The drawing under review shows one solid part. Ordinate dimensions are in mm from its lowest x, y, z. Coordinates: 2 decimals unless noted, no trailing zeros. Write each loop counter-clockwise with the first axis right and the second up, starting at its lowest first coordinate (ties: lowest second). Pieces come first, ordered by that corner, then holes. Notation, with made-up numbers: (40.5, -5.75) - (91.5, -5.75) arc R8 ccw to (91.5, 3.25) - close; hole circle Ø11 at (23, 58.5). An arc over 180 degrees is marked (long way). Use a Markdown table: item, result.
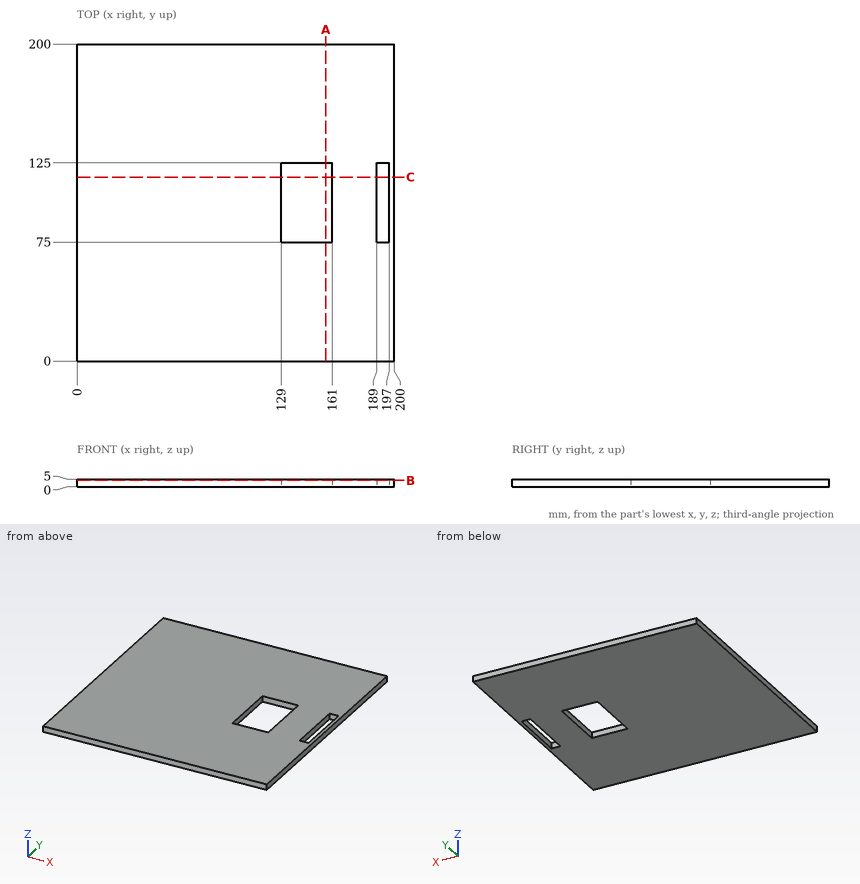
(1) For L1, parallel to X at y = 123, z = 3.65; L2, parallel to Y at x = 149, z = 4.4, list the stretches that pass through material, from the lowest coordinate up. Write a range as from..to.
Determined:
| item | result |
|---|---|
| L1 | 0..129, 161..189, 197..200 |
| L2 | 0..75, 125..200 |
(2) Take a section at C-C on y = 116. Write out the cut boundary in (x, z), and give its area (3 significant figures).
Determined:
| item | result |
|---|---|
| outline | (0, 0) - (129, 0) - (129, 5) - (0, 5) - close; (161, 0) - (189, 0) - (189, 5) - (161, 5) - close; (197, 0) - (200, 0) - (200, 5) - (197, 5) - close |
| area | 800 mm2 |
(3) For pin 1 (2.5 mm diameter, centred on x = 192, z = 1.5, fed in from -Y), flat-tipped, find the tip position at first contact; note if it passes through.
Determined:
| item | result |
|---|---|
| pin 1 | y = 0 |
(4) Take a section at B-B on z = 4.15. Write out the cut boundary in (x, y).
Determined:
| item | result |
|---|---|
| outline | (0, 0) - (200, 0) - (200, 200) - (0, 200) - close; hole (129, 75) - (161, 75) - (161, 125) - (129, 125) - close; hole (189, 75) - (197, 75) - (197, 125) - (189, 125) - close |
(5) Take a section at A-A on x = 157. Write out the cut boundary in (y, z).
Determined:
| item | result |
|---|---|
| outline | (0, 0) - (75, 0) - (75, 5) - (0, 5) - close; (125, 0) - (200, 0) - (200, 5) - (125, 5) - close |
